Model file for the job. Use its own axes, mm. Give positions to 0.01 mm unless a question says otherwise; leave off trailing zeros. Loops run counter-clockwise (first coordinate to the right, second up) from the corner with the lowest first, then second, coordinate; pieces in that order, holes last. Notation, with made-up numbers: M 30.5,68.25 L 44.5,68.25 A30 cw 44.5,106.25 Z; hole C -34.75,14 d6. An arc over 180 degrees is marked long. Use CSV: the item, a comma, the result in double quotes. Start each with the question number.
(1) Flat gauge pins, fed straight in: P1, Ø6.5, axis at x = 185.5, y = 70, coming from the +Z side; P2, Ø3, axis at x = 182.75, y = 8.25, coming from the -Z side; P3, Ø2.5, axis at x = 8.25, y = 106.75, coming from the +Z side; P4, Ø2, axis at x = 55.5, z = 7.5, coming from the -Y side. Where does each tip first touch, or does it go through?
(2) Wall check: line 1 along Y through (x, z) = (182.75, 4.95); line 2 along Y through (x, z) = (8.25, 1.3); line 3 along Y through (x, z) = (150.5, 0.5). Give the ranges that are in metal, low to high. Write a range as from..to.
(3) Slice it at B-B on x = 18. List the corners of the cut face in (y, z), and give its area (3 significant figures).
(4) Slice it at A-A on y = 99.5. List the corners of the cut face in (x, z), and give its area (3 significant figures).
Autodesk Fusion 360 part; units mm, degrees
sketch "sketch_ecran_base" plane through (0, 0, 0) normal (0, 0, 1) x (1, 0, 0)
  line L0 (5, 0) -> (186, 0)
  line L1 (191, 5) -> (191, 110)
  line L2 (186, 115) -> (5, 115)
  line L3 (0, 110) -> (0, 5)
  arc A0 (5, 115) -> (0, 110) centre (5, 110) ccw
  arc A1 (191, 110) -> (186, 115) centre (186, 110) ccw
  arc A2 (186, 0) -> (191, 5) centre (186, 5) ccw
  arc A3 (0, 5) -> (5, 0) centre (5, 5) ccw
  line L4 (6.5, 111.5) -> (184.5, 111.5)
  line L5 (187, 109) -> (187, 6)
  line L6 (184.5, 3.5) -> (6.5, 3.5)
  line L7 (4, 6) -> (4, 109)
  arc A4 (6.5, 111.5) -> (4, 109) centre (6.5, 109) ccw
  arc A5 (187, 109) -> (184.5, 111.5) centre (184.5, 109) ccw
  arc A6 (184.5, 3.5) -> (187, 6) centre (184.5, 6) ccw
  arc A7 (4, 6) -> (6.5, 3.5) centre (6.5, 6) ccw
  point P0 (191, 0)
  point P1 (0, 115)
  point P2 (4, 111.5)
  point P3 (187, 111.5)
  point P4 (4, 3.5)
  dimension "d1" = 191
  dimension "d2" = 115
  dimension "d3" = 5
  dimension "d4" = 5
  dimension "d5" = 183
  dimension "d6" = 108
  dimension "d7" = 2.5
  dimension "d8" = 2.5
  dimension "d9" = 4
  dimension "d10" = 3.5
extrude "Extrude1" add sketch "sketch_ecran_base" along normal blind 15 contours L0 L1 L2 L3 A0 A1 A2 A3 | L4 L5 L6 L7 A4 A5 A6 A7 makes body 1
extrude "Extrude2" add sketch "sketch_ecran_base" along normal blind 0.4 from surface at 15 contours L4 L5 L6 L7 A4 A5 A6 A7 bodies 1
sketch "sketch_ecran_sides" plane through (0, 0, 0) normal (0, -1, 0) x (1, 0, 0)
  line L0 (5, 0) -> (186, 0)
  line L1 (186, 0) -> (186, 15)
  line L2 (186, 15) -> (5, 15)
  line L3 (5, 15) -> (5, 0)
  line L4 (95.5, 15) -> (95.5, 7) construction
  arc A0 (186, 0) -> (5, 0) centre (95.5, -581.5179) ccw
  dimension "d16" = 8
extrude "Extrude3" cut sketch "sketch_ecran_sides" against normal blind 125 contours L0 A0 bodies 1
chamfer "Chamfer1" distance 1.3 distance2 1.8 8 edges at (0, 57.5, 15) (1.4645, 1.4645, 15) (95.5, 0, 15) (189.5355, 1.4645, 15) (191, 57.5, 15) (189.5355, 113.5355, 15) (95.5, 115, 15) (1.4645, 113.5355, 15) measured on face at (189.6667, 74.6667, 15) measured on face at (189.6667, 74.6667, 15) measured on face at (189.6667, 74.6667, 15) measured on face at (189.6667, 74.6667, 15) measured on face at (189.6667, 74.6667, 15) measured on face at (189.6667, 74.6667, 15) measured on face at (189.6667, 74.6667, 15) measured on face at (189.6667, 74.6667, 15) on bodies 1
sketch "sketch_backplate_base" plane through (0, 0, 0) normal (0, 0, 1) x (1, 0, 0)
  line L0 (5, 0) -> (186, 0)
  line L1 (191, 5) -> (191, 110)
  line L2 (186, 115) -> (5, 115)
  line L3 (0, 110) -> (0, 5)
  circle A0 centre (8.25, 106.75) radius 3.25
  circle A1 centre (8.25, 106.75) radius 2
  circle A2 centre (8.25, 106.75) radius 1
  line L4 (95.5, 115) -> (95.5, 0) construction
  line L5 (0, 57.5) -> (191, 57.5) construction
  circle A3 centre (182.75, 106.75) radius 3.25
  circle A4 centre (182.75, 106.75) radius 2
  circle A5 centre (182.75, 106.75) radius 1
  circle A6 centre (8.25, 8.25) radius 3.25
  circle A7 centre (8.25, 8.25) radius 2
  circle A8 centre (8.25, 8.25) radius 1
  circle A9 centre (182.75, 8.25) radius 3.25
  circle A10 centre (182.75, 8.25) radius 2
  circle A11 centre (182.75, 8.25) radius 1
  arc A12 (5, 115) -> (0, 110) centre (5, 110) ccw
  arc A13 (191, 110) -> (186, 115) centre (186, 110) ccw
  arc A14 (186, 0) -> (191, 5) centre (186, 5) ccw
  arc A15 (0, 5) -> (5, 0) centre (5, 5) ccw
  line L6 (1.4, 110) -> (1.4, 5)
  arc A16 (1.4, 5) -> (5, 1.4) centre (5, 5) ccw
  line L7 (5, 1.4) -> (186, 1.4)
  arc A17 (186, 1.4) -> (189.6, 5) centre (186, 5) ccw
  line L8 (189.6, 5) -> (189.6, 110)
  arc A18 (189.6, 110) -> (186, 113.6) centre (186, 110) ccw
  line L9 (186, 113.6) -> (5, 113.6)
  arc A19 (5, 113.6) -> (1.4, 110) centre (5, 110) ccw
  line L10 (5, 2.8) -> (186, 2.8)
  arc A20 (186, 2.8) -> (188.2, 5) centre (186, 5) ccw
  line L11 (188.2, 5) -> (188.2, 110)
  arc A21 (188.2, 110) -> (186, 112.2) centre (186, 110) ccw
  line L12 (186, 112.2) -> (5, 112.2)
  arc A22 (5, 112.2) -> (2.8, 110) centre (5, 110) ccw
  line L13 (2.8, 110) -> (2.8, 5)
  arc A23 (2.8, 5) -> (5, 2.8) centre (5, 5) ccw
  line L14 (13, 102.5) -> (178, 102.5)
  line L15 (178, 102.5) -> (178, 12.5)
  line L16 (178, 12.5) -> (13, 12.5)
  line L17 (13, 12.5) -> (13, 102.5)
  point P0 (191, 0)
  point P1 (0, 115)
  point P2 (13, 57.5)
  point P3 (178, 57.5)
  point P4 (95.5, 102.5)
  dimension "d21" = 191
  dimension "d22" = 115
  dimension "d23" = 6.5
  dimension "d24" = 8.25
  dimension "d25" = 8.25
  dimension "d26" = 4
  dimension "d27" = 2
  dimension "d28" = 5
  dimension "d29" = -1.4
  dimension "d30" = -2.8
  dimension "d57" = 165
  dimension "d58" = 90
sketch "sketch_backplate_side" plane through (0, 0, 0) normal (0, 1, 0) x (1, 0, 0)
  line L0 (0, 0) -> (191, 0)
  line L1 (95.5, 0) -> (95.5, -11.2) construction
  line L2 (0, 0) -> (0, -2.4)
  line L3 (0, -2.4) -> (8.25, -2.4)
  line L4 (8.25, 0) -> (8.25, -2.4)
  line L5 (0, -2.4) -> (0, -3.9)
  line L6 (0, -3.9) -> (8.25, -3.9)
  line L7 (8.25, -2.4) -> (8.25, -3.9)
  line L8 (191, -3.9) -> (182.75, -3.9)
  line L9 (191, -2.4) -> (182.75, -2.4)
  line L10 (191, 0) -> (191, -2.4)
  line L11 (191, -2.4) -> (191, -3.9)
  arc A0 (8.25, -2.4) -> (182.75, -2.4) centre (95.5, 562.3517) ccw
  arc A1 (8.25, -3.9) -> (182.75, -3.9) centre (95.5, 513.8584) ccw
  line L12 (182.75, 0) -> (182.75, -2.4)
  line L13 (182.75, -2.4) -> (182.75, -3.9)
  point P0 (8.25, 0)
  point P1 (182.75, 0)
  point P2 (95.5, -9.1)
  dimension "d31" = 191
  dimension "d32" = 8.25
  dimension "d33" = 11.2
  dimension "d34" = 2.4
  dimension "d35" = 1.5
  dimension "d36" = 9.1
extrude "Extrude4" add sketch "sketch_backplate_base" along normal blind 3.9 separate body contours L6 A16 L7 A17 L8 A18 L9 A19 makes body 2
extrude "Extrude5" add sketch "sketch_backplate_base" along normal blind 2.4 contours L0 L1 L2 L3 A12 A13 A14 A15 | L10 A20 L11 A21 L12 A22 L13 A23 bodies 2
extrude "Extrude6" add sketch "sketch_backplate_side" along normal blind 2.8 contours L0 L4 A0 L12 bodies 2
extrude "Extrude7" add sketch "sketch_backplate_side" against normal blind 1.4 from surface at 2.8 contours L7 A0 A1 L13 bodies 2
extrude "Extrude8" add sketch "sketch_backplate_side" against normal blind 2.8 from surface at 115 contours L0 L4 A0 L12 | L7 A0 A1 L13 bodies 2
extrude "Extrude9" cut sketch "sketch_backplate_side" against normal blind 1.4 from surface at 115 contours L7 A0 A1 L13 bodies 2
extrude "Extrude10" add sketch "sketch_backplate_base" along normal blind 5.8 contours A0 | A3 | A6 | A9 bodies 2
extrude "Extrude11" add sketch "sketch_backplate_base" against normal blind 1.2 from surface at 5.8 contours A1 | A4 | A7 | A10 bodies 2
hidden bodies 1
equation "d9 = ( ( 191 - 183 ) / 2 ) * 1 mm"
equation "d10 = ( ( 115 - 108 ) / 2 ) * 1 mm"
equation "d24 = 5 mm + ( ( 6.5 / 2 ) * 1 mm )"
equation "d25 = 5 mm + ( ( 6.5 / 2 ) * 1 mm )"
equation "d32 = 5 mm + ( ( 6.5 / 2 ) * 1 mm )"
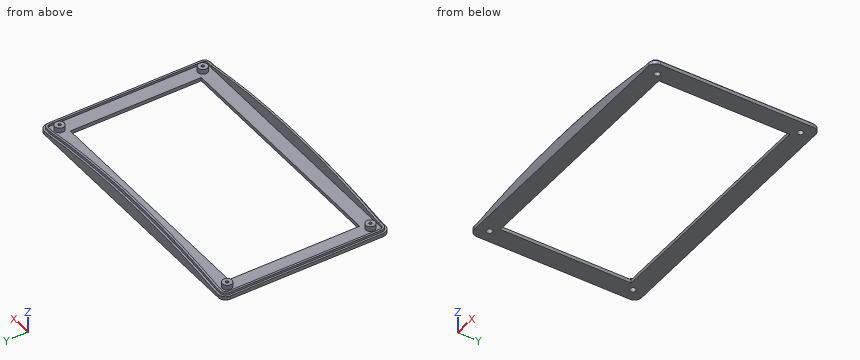
Reply:
1,P1,"stops at z = 3.9"
1,P2,"stops at z = 4.6"
1,P3,"stops at z = 5.8"
1,P4,"stops at y = 0"
2,line 1,"y = 5..7.25, 9.25..11.5, 103.5..105.75, 107.75..110"
2,line 2,"y = 0..6.25, 10.25..104.75, 108.75..115"
2,line 3,"y = 0..12.5, 102.5..115"
3,outline,"M 0,0 L 12.5,0 L 12.5,2.4 L 2.8,2.4 L 2.8,5.45 L 1.4,5.45 L 1.4,3.82 L 0,3.82 Z; M 102.5,0 L 115,0 L 115,3.82 L 113.6,3.82 L 113.6,5.45 L 112.2,5.45 L 112.2,2.4 L 102.5,2.4 Z"
3,area,"72.5 mm^2"
4,outline,"M 0,0 L 13,0 L 13,2.4 L 2.8,2.4 L 2.8,3.9 L 1.4,3.9 L 1.4,2.4 L 0,2.4 Z; M 178,0 L 191,0 L 191,2.4 L 189.6,2.4 L 189.6,3.9 L 188.2,3.9 L 188.2,2.4 L 178,2.4 Z"
4,area,"66.6 mm^2"
